The figure shows three views and two pictorial views of one solid part (mm, origin at its lowest corner). Answer the questions. A direction names the side the tool comes from. Coordinates: 2 decimals unless noted, no trailing zeros. Loops run counter-clockwise (first coordinate to the right, second up) from the corner with the lowest first, then second, coordinate; pieces in that order, holes last. Notation, with made-up numbers: M -7.75,-19 L 6.25,-19 A15 cw 6.25,-11 Z; hole C -32,0.5 d7. An arc over 180 degrees is marked long. Return JSON: item names as keys, results as strings. Group by question number.
1. Section B-B (z = 12) is taken. Write down the section's boundary in (x, y) (1 decimal).
2. The mould has two halves that part along Y. Classify the marked faces 1, 2, 3 and 4: pulls with the +Y half, pulls with the -Y half, needs draft (parallel to the pull), parting line crosses it, or undercut.
3. Given P1, Ø3, axis at x = 15.11, z = 9, coming from the -Y side; P2, Ø2, axis at y = 39.23, z = 9, coming from the +X side (1 decimal); P3, Ø5, axis at x = 2.5, z = 5, coming from the -Y side; P4, Ø3, axis at y = 22.5, z = 16, coming from the -X side (1 decimal), each flat-ended and moving along its own axis, determine where each tip first touches the part or whether it passes through.
4. Which of the six approach directions +Z, -Z, +X, -X, +Y, -Y give full straight-line access (tool end or side, diameter ignored) to the marked faces 5, 6, 7 and 8?
5. Section D-D (z = 9) is taken. Count the separate pieces of the cut face and the enclosed holes in it.
6. Straight lines are drawn through the part: L1, parallel to X at y = 0.45, z = 9; L2, parallel to Y at x = 8.6, z = 9; L3, parallel to Z at x = 8.25, y = 17. For each, find the intervals that lie inside material, in ascending order. Write a range as from..to.
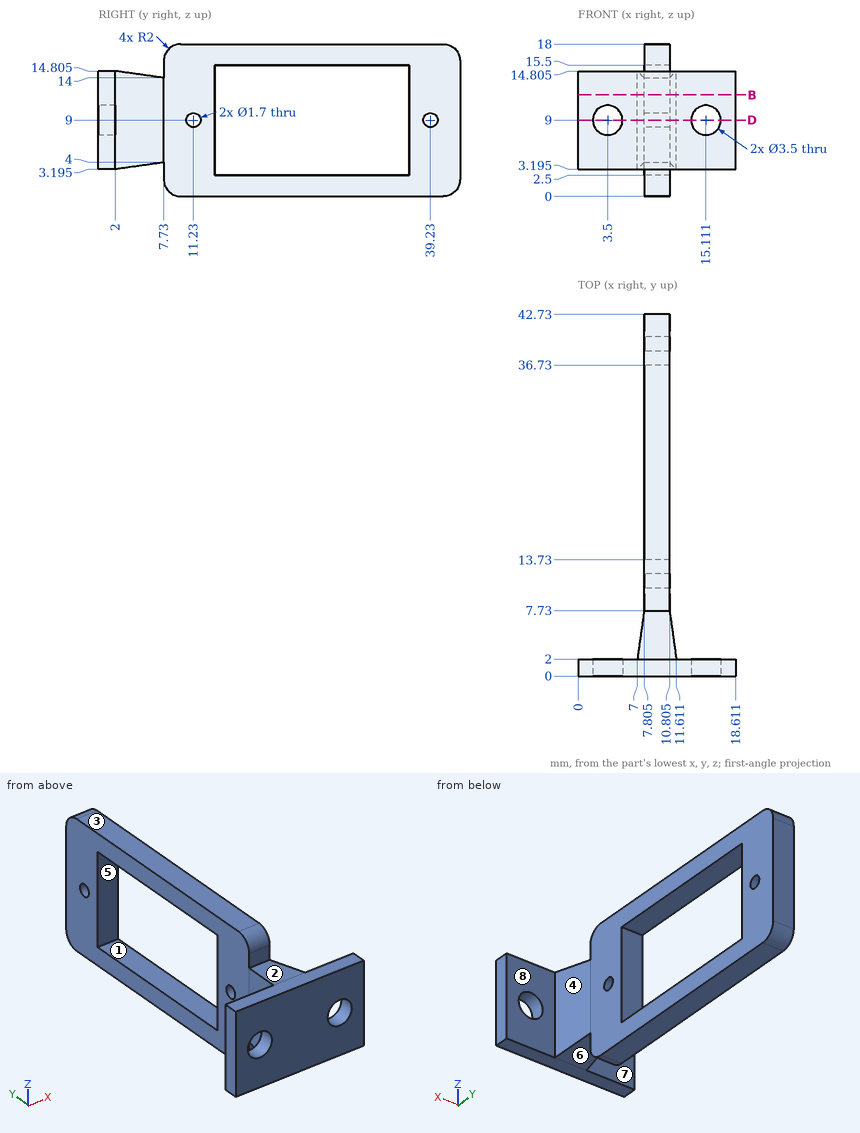
Worked out:
{
 "1": {"outline": "M 0,0 L 18.6,0 L 18.6,2 L 11.6,2 L 10.8,7.7 L 10.8,13.7 L 7.8,13.7 L 7.8,7.7 L 7,2 L 0,2 Z; M 7.8,36.7 L 10.8,36.7 L 10.8,42.7 L 7.8,42.7 Z"},
 "2": {"face 1": "undercut", "face 2": "undercut", "face 3": "needs draft", "face 4": "pulls with the +Y half"},
 "3": {"P1": "through", "P2": "x = 10.8", "P3": "y = 0", "P4": "x = 7.8"},
 "4": {"face 5": "+X, -X", "face 6": "-Z, +X, -X", "face 7": "+Z, -Z, -X, +Y", "face 8": "+Z, -Z, +X, +Y"},
 "5": {"separate pieces": "6", "enclosed holes": "0"},
 "6": {"L1": "0..1.75, 5.25..13.36, 16.86..18.61", "L2": "0..10.38, 12.08..13.73, 36.73..38.38, 40.08..42.73", "L3": "0..2.5, 15.5..18"}
}
